Work out the finished part from the listing and answer in its coordinate system (mm). A direction names the side the tool comes from. Round coordinates to 2 decimals unless told otherwise and drop trailing zeros. Loops run counter-clockwise (first coordinate to the right, second up) from the corner with the lowest first, then second, coordinate; pieces in that order, holes last. Notation, with made-up numbers: (1, 48.5) - (53, 48.5) arc R30 ccw to (53, 70.5) - close; hole circle Ø11 at (9, 65). An arc over 180 degrees is marked (long way). Answer as CSV lines item,"result". Start each with the question number.
Q1. Section D-D on z = 96 is taken. Write down the section's boundary in (x, y).
Q2. Each of these flat-tipped pins is pushed along its axis until it touches: pin 1 Ø1.5 at (x, z) = (18, 20) entering from +Y; pin 2 Ø1.5 at (x, z) = (69.5, 15.5) entering from -Y; pin 3 Ø18 at (y, z) = (15, 98) entering from +X; pin 4 Ø1 at (x, y) = (67.5, 64) entering from +Z. Where does it stop, or does it pass through?
Q3. Section A-A on x = 50 is taken. Write down the section's boundary in (y, z).
Q4. Section B-B on z = 112 is taken. Write down the section's boundary in (x, y).
Q5. Section C-C on y = 46.5 is taken. Write down the section's boundary in (x, z), then the cut area to 3 significant figures.
Q6. For faces 1 (the face through (15, 30, 74)), 2 (the face through (5.703, 73.986, 76.05)), determine the directions among +Z, -Z, +X, -X, +Y, -Y from which every point of the face is accessible in a straight line to the end or side of a thin tool.
Q7. The mould has two halves that part along Y. Classify faces 3 (the face through (7.395, 40.208, 92.113)), 4 (the face through (16, 63, 76)), 5 (the face through (31, 67, 150)): +Y half, -Y half, draft (parallel to the pull), parting line (faces both ways), or undercut.
Q8. Straight lines are drawn through the part: L1, parallel to Z at x = 50, y = 73; L2, parallel to Y at x = 48, z = 64.5; L3, parallel to X at y = 11, z = 26. For each, find the intervals that lie inside material, in ascending order. Write a range as [from, to].
```python
from build123d import *

# Parameters (mm, degrees)
F1_DEPTH = 150
F2_R     = 20
F3_R     = 5
F4_R     = 10
F5_DEPTH = 80.001
F6_R     = 10
F7_DEPTH = 80.001


with BuildPart() as f1:
    # F0 (on Top) → F1 (new body)
    with BuildSketch(Plane.XY):
        Polygon((0, 80), (0, 0), (15, 0), (15, 65), (80, 65), (80, 80), align=None)
    extrude(amount=F1_DEPTH)

    # F2
    f2_edges = [f1.edges().sort_by_distance(p)[0] for p in [
        (0, 80, 75),
    ]]
    fillet(f2_edges, radius=F2_R)

    # F3
    f3_edges = [f1.edges().sort_by_distance(p)[0] for p in [
        (15, 65, 75),
    ]]
    fillet(f3_edges, radius=F3_R)

    # F4 (on face) → F5 (cut, through all)
    with BuildSketch(Plane(origin=(0, 0, 0), x_dir=(0, -1, 0), z_dir=(-1, 0, 0))):
        with Locations((-38.906008, 82.198426)):
            Circle(F4_R)
    extrude(amount=-F5_DEPTH, mode=Mode.SUBTRACT)

    # F6 (on face) → F7 (cut, through all)
    with BuildSketch(Plane(origin=(0, 80, 0), x_dir=(-1, 0, 0), z_dir=(0, 1, 0))):
        with Locations((-50, 87.686576)):
            Circle(F6_R)
    extrude(amount=-F7_DEPTH, mode=Mode.SUBTRACT)


solid = f1.part
```
Findings:
1,outline,"(0, 0) - (15, 0) - (15, 60) arc R5 cw to (20, 65) - (44.44, 65) - (44.44, 80) - (20, 80) arc R20 ccw to (0, 60) - close; (55.56, 65) - (80, 65) - (80, 80) - (55.56, 80) - close"
2,pin 1,"stops at y = 79.96"
2,pin 2,"stops at y = 65"
2,pin 3,"stops at x = 15"
2,pin 4,"passes through"
3,outline,"(65, 0) - (80, 0) - (80, 77.69) - (65, 77.69) - close; (65, 97.69) - (80, 97.69) - (80, 150) - (65, 150) - close"
4,outline,"(0, 0) - (15, 0) - (15, 60) arc R5 cw to (20, 65) - (80, 65) - (80, 80) - (20, 80) arc R20 ccw to (0, 60) - close"
5,outline,"(0, 0) - (15, 0) - (15, 75.69) - (0, 75.69) - close; (0, 88.7) - (15, 88.7) - (15, 150) - (0, 150) - close"
5,area,"2,050 mm^2"
6,face 1,"+Z, -Z, +X, -Y"
6,face 2,"+Z, -Z, -X, +Y"
7,face 3,"undercut"
7,face 4,"-Y half"
7,face 5,"draft"
8,L1,"z = [0, 77.69], [97.69, 150]"
8,L2,"y = [65, 80]"
8,L3,"x = [0, 15]"
